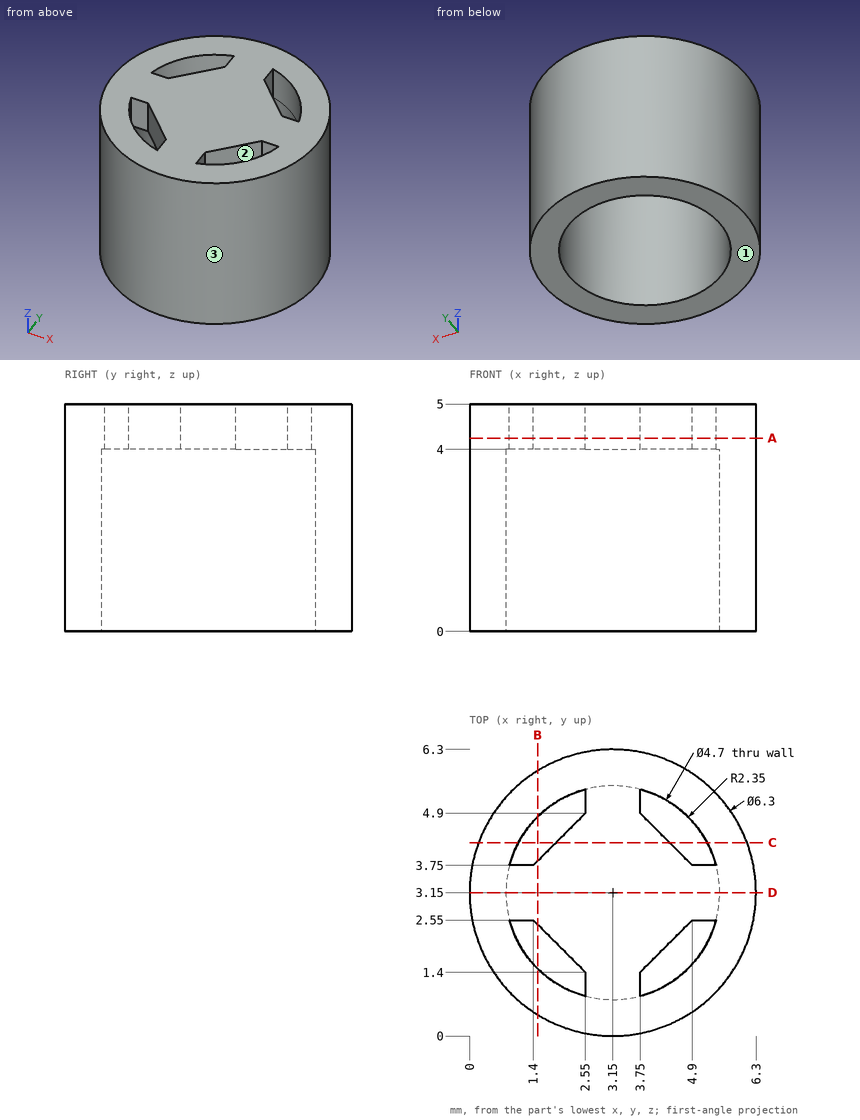
Could you check a few things on this drawing? It's one solid part, dimensions in mm from its lowest x, y, z. Round coordinates to 2 decimals unless told otherwise and drop trailing zeros. Loops run counter-clockwise (first coordinate to the right, second up) from the corner with the lowest first, then second, coordinate; pieces in that order, holes last. Notation, with made-up numbers: (18, 81.5) -> (31, 81.5) arc R22 ccw to (31, 106.5) -> close; hole circle Ø4 at (34, -20.5). An arc over 180 degrees is marked (long way). One line per item, written item: value. Start each with the question number.
1. If we section it at B-B, the plane x = 1.5: Write out the boundary of the cut face in (y, z).
2. If we section it at C-C, the plane y = 4.25: Write out the boundary of the cut face in (x, z), then the cut area to 3 significant figures.
3. If we section it at A-A, the plane z = 4.25: Write out the boundary of the cut face in (x, y).
4. If we section it at D-D, the plane y = 3.15: Write out the boundary of the cut face in (x, z), then the cut area to 3 significant figures.
5. If I drill on probe 1 along Y at (x, z) = (3.15, 0.95); probe 2 along X at (y, z) = (4.25, 4.8); probe 3 along Z at (x, y) = (4.5, 4), over which ranges is the centre line in solid material (lowest first)?
6. If we mould it in two halves opening along Y, with no side actions, what happens to the marked faces 1, 2 and 3? For each: pulls with the +Y half, pulls with the -Y half, needs draft (parallel to the pull), parting line crosses it, or undercut.
7. For pin 1 (2 mm diameter, centred on x = 1, z = 2, fed in from -Y); pin 2 (2 mm diameter, centred on y = 4, z = 1.5, fed in from -X); pin 3 (1.4 mm diameter, centred on x = 4, y = 4, fed in from -Z), each with a flat end and sliding along its axis, tell me the tip position at first contact or that it passes through.
Calculated:
1. outline: (0.47, 0) -> (1.48, 0) -> (1.48, 5) -> (0.47, 5) -> close; (2.45, 4) -> (3.85, 4) -> (3.85, 5) -> (2.45, 5) -> close; (4.82, 0) -> (5.83, 0) -> (5.83, 5) -> (4.82, 5) -> close
2. outline: (0.2, 0) -> (1.07, 0) -> (1.07, 5) -> (0.2, 5) -> close; (1.9, 4) -> (4.4, 4) -> (4.4, 5) -> (1.9, 5) -> close; (5.23, 0) -> (6.1, 0) -> (6.1, 5) -> (5.23, 5) -> close
2. area: 11.3 mm²
3. outline: circle Ø6.3 at (3.15, 3.15); hole (0.88, 2.55) arc R2.35 ccw to (2.55, 0.88) -> (2.55, 1.4) -> (1.4, 2.55) -> close; hole (0.88, 3.75) -> (1.4, 3.75) -> (2.55, 4.9) -> (2.55, 5.42) arc R2.35 ccw to start; hole (3.75, 0.88) arc R2.35 ccw to (5.42, 2.55) -> (4.9, 2.55) -> (3.75, 1.4) -> close; hole (3.75, 4.9) -> (4.9, 3.75) -> (5.42, 3.75) arc R2.35 ccw to (3.75, 5.42) -> close
4. outline: (0, 0) -> (0.8, 0) -> (0.8, 4) -> (5.5, 4) -> (5.5, 0) -> (6.3, 0) -> (6.3, 5) -> (0, 5) -> close
4. area: 12.7 mm²
5. probe 1: y = 0 to 0.8, 5.5 to 6.3
5. probe 2: x = 0.2 to 1.07, 1.9 to 4.4, 5.23 to 6.1
5. probe 3: z = 4 to 5
6. face 1: needs draft
6. face 2: undercut
6. face 3: parting line crosses it
7. pin 1: stops at y = 0.22
7. pin 2: stops at x = 0
7. pin 3: stops at z = 4
